Design review of the part built by this model. Coordinates are the model's own, in mm. A direction names the side the tool comes from. Give positions to 0.01 mm unless a question says otherwise; leave off trailing zeros. Loops run counter-clockwise (first coordinate to the right, second up) from the corner with the lowest first, then second, coordinate; pieces in that order, holes last.
from build123d import *

# Parameters (mm, degrees)
F0_R     = 12
F1_DEPTH = 31
F2_R     = 10
F3_DEPTH = 11.5
F4_SIZE  = 2


# Not quite as in the source:
# - a pattern or mirror of a feature is missing from the dataset's text; its kind, count and spacing are read off the source's solid


with BuildPart() as f1:
    # F0 (on Top) → F1 (new body, symmetric)
    with BuildSketch(Plane.XY):
        Circle(F0_R)
    extrude(amount=F1_DEPTH, both=True)

    # F2 (on face) → F3 (join)
    with BuildSketch(Plane.XY.offset(31)):
        Circle(F2_R)
    f3 = extrude(amount=F3_DEPTH)

    # F3_copies: F3 across plane
    add(f3.mirror(Plane(origin=(0, 0, 0), x_dir=(-1, 0, 0), z_dir=(0, 0, -1))))

    # F4
    f4_edges = [f1.edges().sort_by_distance(p)[0] for p in [
        (-10, 0, 42.5),
        (-10, 0, -42.5),
    ]]
    chamfer(f4_edges, length=F4_SIZE)


solid = f1.part
Q1. Take a section at D-D (z = 1). Give the boundary of the cut face in (x, y), plus the area to 3 significant figures.
Results:
outline: circle Ø24 at (0, 0)
area: 452 mm2
Q2. Take a section at C-C (z = -32). Give the boundary of the cut face in (x, y), plus the area to 3 significant figures.
Results:
outline: circle Ø20 at (0, 0)
area: 314 mm2
Q3. Wall thickness on line 1 (Z direction, x = -8, y = 6.25); line 2 (Y direction, x = -11, z = -10.5); line 3 (X direction, y = 3.75, z = 6.5): over which ranges is each line inside the solid? List them lowest first.
Results:
line 1: z = -31 to 31
line 2: y = -4.8 to 4.8
line 3: x = -11.4 to 11.4
Q4. Take a section at A-A (x = 0). Give the boundary of the cut face in (y, z), plus the area to 3 significant figures.
Results:
outline: (-12, -31) - (-10, -31) - (-10, -40.5) - (-8, -42.5) - (8, -42.5) - (10, -40.5) - (10, -31) - (12, -31) - (12, 31) - (10, 31) - (10, 40.5) - (8, 42.5) - (-8, 42.5) - (-10, 40.5) - (-10, 31) - (-12, 31) - close
area: 1,940 mm2
Q5. Tool access review of faces 1 (the face through (0, 0, 42.5)), 2 (the face through (-2.17, -9.76, -35.68)), 3 (the face through (-5, 9, 31)): name each direction out of +Z, -Z, +X, -X, +Y, -Y from which nothing blocks a thin tool from reaching the whole face with its end or side.
Results:
face 1: +Z, +X, -X, +Y, -Y
face 2: -Z
face 3: +Z
Q6. Insertion check: pin 1 (8 mm diameter, centred on y = 8, z = 5, fed in from +X); pin 2 (5 mm diameter, centred on x = 7.5, z = -31.5, fed in from -Y); pin 3 (1 mm diameter, centred on y = -8, z = -2.5, fed in from +X); pin 4 (10 mm diameter, centred on x = 1.5, z = 20.5, fed in from +Y). Each pin has a flat end and moves straight along its axis. Give the tip position at first contact, or say it passes through.
Results:
pin 1: stops at x = 11.31
pin 2: stops at y = -10.89
pin 3: stops at x = 9.37
pin 4: stops at y = 12
